from build123d import *

# Parameters (mm, degrees)
SKETCH1_W           = 35.2
SKETCH1_H           = 24.5
SKETCH1_R           = 1.35
BOSS_EXTRUDE1_DEPTH = 1.5
SKETCH2_R           = 1.2
SKETCH2_W           = 5
SKETCH2_H           = 1.5
SKETCH2_W_2         = 14.5
BOSS_EXTRUDE2_DEPTH = 1.5
SKETCH3_R           = 1.2
BOSS_EXTRUDE3_DEPTH = 1.5
CHAMFER1_SIZE       = 1.5


with BuildPart() as part:
    # Sketch1 → Boss-Extrude1 (new body)
    with BuildSketch(Plane(origin=(0, 0, 0), x_dir=(1, 0, 0), z_dir=(0, 1, 0))):
        Rectangle(SKETCH1_W, SKETCH1_H)
        with Locations(Location((-5, 5, 0), (0, 0, 270))):
            Circle(SKETCH1_R, mode=Mode.SUBTRACT)
        with Locations(Location((5, 5, 0), (0, 0, 90))):
            Circle(SKETCH1_R, mode=Mode.SUBTRACT)
        with Locations(Location((-5, -5, 0), (0, 0, 90))):
            Circle(SKETCH1_R, mode=Mode.SUBTRACT)
        with Locations(Location((5, -5, 0), (0, 0, 270))):
            Circle(SKETCH1_R, mode=Mode.SUBTRACT)
    extrude(amount=BOSS_EXTRUDE1_DEPTH)

    # Sketch2 → Boss-Extrude2 (add)
    # profile 1 of 6: a face of its own
    with BuildSketch(Plane(origin=(17.6, 0, 0), x_dir=(0, 0, -1), z_dir=(1, 0, 0))):
        with BuildLine():
            Line((-7.25, 1.5), (-7.25, 3))
            Line((-7.25, 3), (-7.25, 11.51))
            Line((-7.25, 11.51), (-10.25, 11.51))
            ThreePointArc((-10.25, 11.51), (-11.664213562, 10.924213562), (-12.25, 9.51))
            Line((-12.25, 9.51), (-12.25, 1.5))
            Line((-12.25, 1.5), (-7.25, 1.5))
        make_face()
        with Locations((-10.25, 9.51)):
            Circle(SKETCH2_R, mode=Mode.SUBTRACT)
    # profile 2 of 6: a face of its own
    with BuildSketch(Plane(origin=(17.6, 0, 0), x_dir=(0, 0, -1), z_dir=(1, 0, 0))):
        with Locations((-9.75, 0.75)):
            Rectangle(SKETCH2_W, SKETCH2_H)
    # profile 3 of 6: a face of its own
    with BuildSketch(Plane(origin=(17.6, 0, 0), x_dir=(0, 0, -1), z_dir=(1, 0, 0))):
        with Locations((0, 0.75)):
            Rectangle(SKETCH2_W_2, SKETCH2_H)
    # profile 4 of 6: a face of its own
    with BuildSketch(Plane(origin=(17.6, 0, 0), x_dir=(0, 0, -1), z_dir=(1, 0, 0))):
        with Locations((0, 2.25)):
            Rectangle(SKETCH2_W_2, SKETCH2_H)
    # profile 5 of 6: a face of its own
    with BuildSketch(Plane(origin=(17.6, 0, 0), x_dir=(0, 0, -1), z_dir=(1, 0, 0))):
        with Locations((9.75, 0.75)):
            Rectangle(SKETCH2_W, SKETCH2_H)
    # profile 6 of 6: a face of its own
    with BuildSketch(Plane(origin=(17.6, 0, 0), x_dir=(0, 0, -1), z_dir=(1, 0, 0))):
        with BuildLine():
            Line((7.25, 11.51), (7.25, 3))
            Line((7.25, 3), (7.25, 1.5))
            Line((7.25, 1.5), (12.25, 1.5))
            Line((12.25, 1.5), (12.25, 9.51))
            ThreePointArc((12.25, 9.51), (11.664213562, 10.924213562), (10.25, 11.51))
            Line((10.25, 11.51), (7.25, 11.51))
        make_face()
        with Locations((10.25, 9.51)):
            Circle(SKETCH2_R, mode=Mode.SUBTRACT)
    extrude(amount=-BOSS_EXTRUDE2_DEPTH)

    # Sketch3 → Boss-Extrude3 (add)
    with BuildSketch(Plane.ZY.offset(17.6)):
        with BuildLine():
            Line((-12.25, 0), (12.25, 0))
            Line((12.25, 0), (12.25, 5.76))
            ThreePointArc((12.25, 5.76), (11.664213562, 7.174213562), (10.25, 7.76))
            Line((10.25, 7.76), (-10.25, 7.76))
            ThreePointArc((-10.25, 7.76), (-11.664213562, 7.174213562), (-12.25, 5.76))
            Line((-12.25, 5.76), (-12.25, 0))
        make_face()
        with Locations((-10.25, 5.76)):
            Circle(SKETCH3_R, mode=Mode.SUBTRACT)
        with Locations(Location((10.25, 5.76, 0), (0, 0, 180))):
            Circle(SKETCH3_R, mode=Mode.SUBTRACT)
    extrude(amount=-BOSS_EXTRUDE3_DEPTH)

    # Chamfer1
    chamfer1_edges = [part.edges().sort_by_distance(p)[0] for p in [
        (16.1, 1.5, 0),
        (-16.1, 1.5, 0),
    ]]
    chamfer(chamfer1_edges, length=CHAMFER1_SIZE - 0.0001)  # a hair under: the kernel refuses the full size


solid = part.part
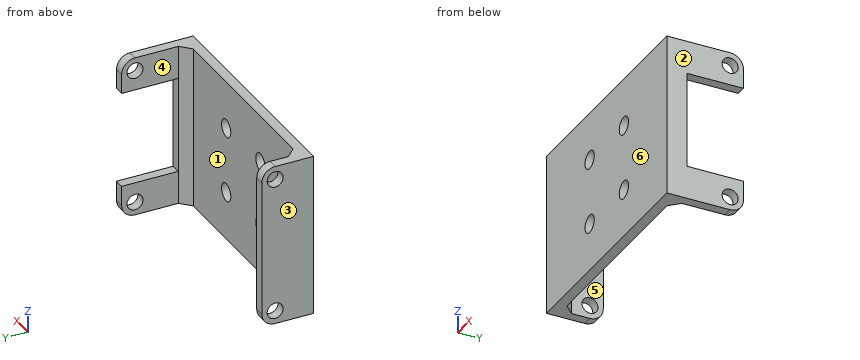
Work out the finished part from the listing and answer in its coordinate system (mm). Face numbers are marked on the shaded views. A direction names the side the tool comes from. Give positions to 0.01 mm unless a question says otherwise; leave off trailing zeros. Write each loop counter-clockwise with the first axis right and the second up, starting at its lowest first coordinate (ties: lowest second). Pieces come first, ordered by that corner, then holes. Notation, with made-up numbers: (85, 4) - (117, 4) arc R14 ccw to (117, 17) - close; hole circle Ø10 at (55.5, -22.5). An arc over 180 degrees is marked (long way). One line per item, written item: value. Start each with the question number.
1. Consider probe 1 along X at (y, z) = (1.15, 5); probe 2 along Y at (x, z) = (16.45, 10.25); probe 3 along Y at (x, z) = (-13, 5). Determine where each line is inside the solid, lowest interval first.
2. Find section A-A (z = -5). State how many separate pieces and enclosed holes the cut face has, then the cut area to 3 significant figures.
3. Given pin 1 (3 mm diameter, centred on x = 12, z = -8, fed in from -Y); pin 2 (0.8 mm diameter, centred on x = 17, z = 3, fed in from +Y); pin 3 (2 mm diameter, centred on x = 5, z = -5, fed in from +Y); pin 4 (1.4 mm diameter, centred on y = 5.76, z = 10.25, fed in from -X), each flat-ended and moving along its own axis, determine where each tip first touches the part or whether it passes through.
4. For a pull along X with two mould halves and no side action, classify the marked faces 1, 2, 3 and 4 as +X half, -X half, draft (parallel to the pull), parting line (faces both ways), or undercut.
5. Find section B-B (y = 1). Write down the section's boundary in (x, z), then the cut area to 4 significant figures.
6. For the marked faces 5 and 6, determine the directions among +Z, -Z, +X, -X, +Y, -Y from which every point of the face is accessible in a straight line to the end or side of a thin tool.
7. Find section C-C (y = 5). Write down the section's boundary in (x, z), then the cut area to 3 significant figures.
Geometry results:
1. probe 1: -17.6 to -6.35, -3.65 to 3.65, 6.35 to 17.6
1. probe 2: 0 to 8.31, 10.71 to 11.51
1. probe 3: 0 to 1.5
2. separate pieces: 3
2. enclosed holes: 0
2. area: 58.6 mm2
3. pin 1: y = 0
3. pin 2: y = 3
3. pin 3: through
3. pin 4: x = 16.1
4. face 1: undercut
4. face 2: +X half
4. face 3: -X half
4. face 4: undercut
5. outline: (-17.6, -12.25) - (17.6, -12.25) - (17.6, 12.25) - (-17.6, 12.25) - close; hole circle Ø2.7 at (-5, -5); hole circle Ø2.7 at (-5, 5); hole circle Ø2.7 at (5, -5); hole circle Ø2.7 at (5, 5)
5. area: 839.5 mm2
6. face 5: +Z, -Z, +Y
6. face 6: +Z, -Z, +X, -X, -Y
7. outline: (-17.6, -12.25) - (-16.1, -12.25) - (-16.1, -11.18) - (-17.6, -11.18) - close; (-17.6, -9.32) - (-16.1, -9.32) - (-16.1, 9.32) - (-17.6, 9.32) - close; (-17.6, 11.18) - (-16.1, 11.18) - (-16.1, 12.25) - (-17.6, 12.25) - close; (16.1, -12.25) - (17.6, -12.25) - (17.6, -7.25) - (16.1, -7.25) - close; (16.1, 7.25) - (17.6, 7.25) - (17.6, 12.25) - (16.1, 12.25) - close
7. area: 46.2 mm2
